Here's the drawing with two shaded views (mm, measured from the low corner). I have some questions. A direction names the side the tool comes from. Give positions to 0.01 mm unless a question says otherwise; leave off trailing zeros. Write each loop counter-clockwise with the first axis right and the second up, starting at its lowest first coordinate (ties: lowest second). Pieces come first, ordered by that corner, then holes. Notation, with made-up numbers: (9.5, 55.25) -> (45.5, 55.25) arc R17 ccw to (45.5, 88.25) -> close; hole circle Ø2 at (-8, 10). An arc over 180 degrees is marked (long way). One line per item, written item: value.
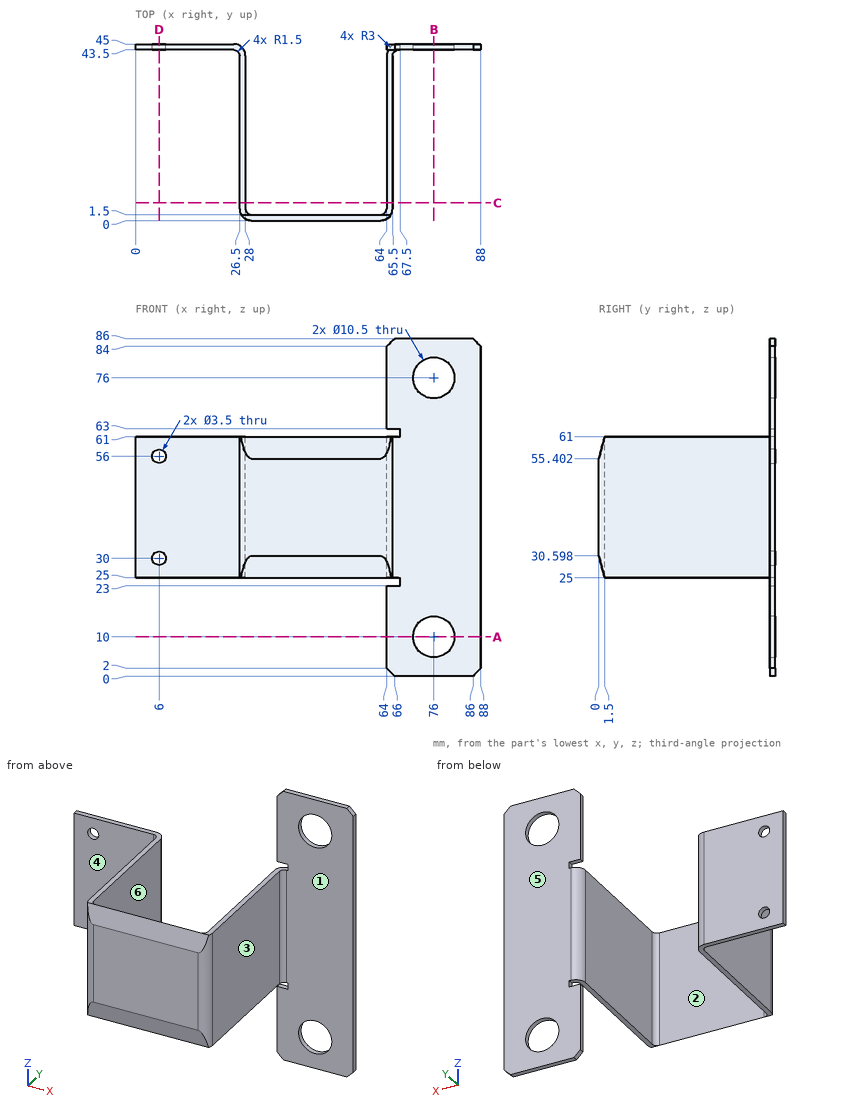
1) If we section it at D-D (x = 6): Write out the boundary of the cut face in (y, z), and give its area (3 significant figures).
Answer list:
outline: (43.5, 25) -> (45, 25) -> (45, 28.25) -> (43.5, 28.25) -> close; (43.5, 31.75) -> (45, 31.75) -> (45, 54.25) -> (43.5, 54.25) -> close; (43.5, 57.75) -> (45, 57.75) -> (45, 61) -> (43.5, 61) -> close
area: 43.5 mm^2
2) Will these pins go through, and if not, where does the flat tip stop? pin 1 (12 mm diameter, centred on x = 76, z = 10, fed in from -Y); pin 2 (18 mm diameter, centred on y = 20, z = 46, fed in from +X); pin 3 (2.5 mm diameter, centred on x = 66, y = 22, fed in from -Z).
Answer list:
pin 1: stops at y = 43.5
pin 2: stops at x = 65.5
pin 3: stops at z = 25
3) We'd pull the mould along X, two halves only. Please class the marked faces 1, 2 and 3: released by +X, released by -X, zero draft, split by the parting line, or undercut.
Answer list:
face 1: zero draft
face 2: undercut
face 3: released by +X
4) If we section it at B-B (x = 76): Write out the boundary of the cut face in (y, z), and give its area (3 significant figures).
Answer list:
outline: (43.5, 0) -> (45, 0) -> (45, 4.75) -> (43.5, 4.75) -> close; (43.5, 15.25) -> (45, 15.25) -> (45, 70.75) -> (43.5, 70.75) -> close; (43.5, 81.25) -> (45, 81.25) -> (45, 86) -> (43.5, 86) -> close
area: 97.5 mm^2
5) If we section it at C-C (y = 4.5): Write out the boundary of the cut face in (x, z), and give its area (3 significant figures).
Answer list:
outline: (26.5, 25) -> (28, 25) -> (28, 61) -> (26.5, 61) -> close; (64, 25) -> (65.5, 25) -> (65.5, 61) -> (64, 61) -> close
area: 108 mm^2
6) If we section it at A-A (z = 10): Write out the boundary of the cut face in (x, y).
Answer list:
outline: (64, 43.5) -> (70.75, 43.5) -> (70.75, 45) -> (64, 45) -> close; (81.25, 43.5) -> (88, 43.5) -> (88, 45) -> (81.25, 45) -> close
7) For the marked faces 4, 5 and 6, which set-ups out of +Z, -Z, +X, -X, +Y, -Y let a thin tool reach every point of the face, with its end or its side?
Answer list:
face 4: +Z, -Z, -X, -Y
face 5: +Z, -Z, +X, -X, +Y
face 6: +Z, -Z, +Y
8) I need wall thicknesses on L1, parallel to X at y = 35, z = 29.5; L2, parallel to X at y = 44.7, z = 76; L3, parallel to Y at x = 81.5, z = 17.5. Which ranges of each line are inside material? Lowest first, please.
Answer list:
L1: x = 26.5 to 28, 64 to 65.5
L2: x = 64 to 70.75, 81.25 to 88
L3: y = 43.5 to 45
